Model file for the job. Use its own axes, mm. Face numbers are marked on the shaded views. A direction names the side the tool comes from. Round coordinates to 2 decimals unless told otherwise and drop trailing zeros. Order: outer loops, then holes, each group sorted by start corner. A loop starts at its lowest first (then second) coordinate and runs counter-clockwise, first axis right, second up. Notation, with made-up numbers: (18.25, 63) -> (38.25, 63) arc R12 cw to (38.25, 77) -> close; hole circle Ø4 at (20, 48). An arc over 180 degrees is marked (long way). Use CSV: the item, a comma, the result in double quotes.
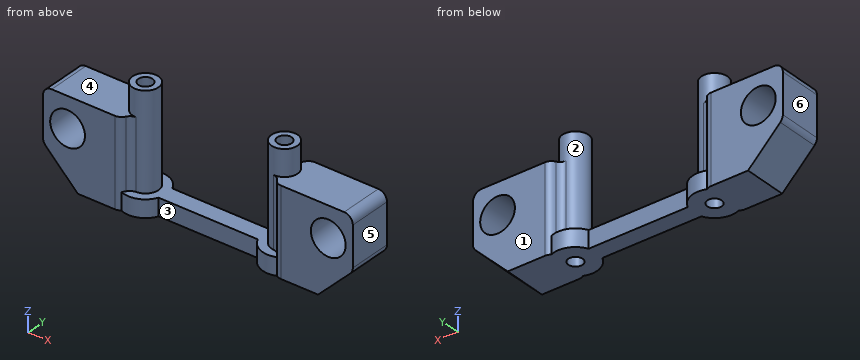
Autodesk Inventor part; units mm, degrees
ref_plane "YZ Plane" through (0, 0, 0) normal (1, 0, 0) x (0, 1, 0)
ref_plane "XZ Plane" through (0, 0, 0) normal (0, 1, 0) x (-1, 0, 0)
ref_plane "XY Plane" through (0, 0, 0) normal (0, 0, 1) x (1, 0, 0)
sketch "Sketch1" plane through (0, 0, 0) normal (0, 0, 1) x (1, 0, 0)
  circle A0 centre (0, 0) radius 1.65
  circle A1 centre (0, 0) radius 3
  circle A2 centre (32, 0) radius 1.65
  circle A3 centre (32, 0) radius 3
  dimension "d0" = 3.3
  dimension "d1" = 6
  dimension "d22" = 32
extrude "Extrusion1" add sketch "Sketch1" along normal blind 26
sketch "Sketch2" plane through (0, 0, 0) normal (0, 0, -1) x (-1, 0, 0)
  circle A0 centre (0, 0) radius 3
  circle A1 centre (0, 0) radius 5
  circle A2 centre (-32, 0) radius 1.65
  circle A3 centre (-32, 0) radius 5
  circle A4 centre (0, 0) radius 1.65 construction
  line L0 (-30.35, 2) -> (-1.65, 2)
  line L1 (-1.65, 2) -> (-1.65, -2)
  line L2 (-1.65, -2) -> (-30.35, -2)
  line L3 (-30.35, -2) -> (-30.35, 2)
  point P0 (-1.65, 0)
  dimension "d4" = 10
  dimension "d7" = 4
extrude "Extrusion2" add sketch "Sketch2" against normal blind 4 contours A0 L0 A1 L2 | L0 L1 L2 A0 | A0 L2 A1 L0 | A1 L2 A3 L0 | L0 L3 L2 A3 | A3 L2 L3 L0 picked at (-2.1, 0)
sketch "Sketch3" plane through (0, 0, 0) normal (0, 0, -1) x (-1, 0, 0)
  line L0 (-51.65, -5) -> (-33.65, -5)
  line L1 (-33.65, -5) -> (-33.65, 5)
  line L2 (-33.65, 5) -> (-51.65, 5)
  line L3 (-51.65, 5) -> (-51.65, -5)
  line L4 (1.65, 5) -> (19.65, 5)
  line L5 (19.65, 5) -> (19.65, -5)
  line L6 (19.65, -5) -> (1.65, -5)
  line L7 (1.65, -5) -> (1.65, 5)
  circle A0 centre (0, 0) radius 1.65 construction
  circle A1 centre (-32, 0) radius 1.65 construction
  arc A2 (-27.4174, 2) -> (-27.4174, -2) centre (-32, 0) ccw construction
  arc A3 (-4.5826, -2) -> (-4.5826, 2) centre (0, 0) ccw construction
  point P0 (-33.65, 0)
  point P1 (1.65, 0)
  dimension "d8" = 18
  dimension "d10" = 18
extrude "Extrusion3" add sketch "Sketch3" against normal blind 20
sketch "Sketch4" plane through (33.65, 5, 0) normal (0, 1, 0) x (1, 0, 0)
  circle A0 centre (-47.65, -13) radius 4
  circle A1 centre (12.35, -13) radius 4
  line L0 (-35.3, -20) -> (-53.3, -20)
  line L1 (18, -20) -> (0, -20)
  line L2 (-35.3, 0) -> (-53.3, 0)
  line L3 (18, 0) -> (18, -20)
  line L4 (-53.3, 0) -> (-53.3, -20)
  point P0 (-33.65, 0)
  point P1 (-44.3, -20)
  point P2 (9, -20)
  dimension "d13" = 8
  dimension "d14" = 8
  dimension "d15" = 13
  dimension "d23" = 60
  dimension "d24" = 5.65
  dimension "d25" = 5.65
extrude "Extrusion4" cut sketch "Sketch4" against normal blind 20
chamfer "Chamfer1" distance 8 angle 45 2 edges at (51.65, 0, 0) (-19.65, 0, 0)
fillet "Fillet1" radius 2 12 edges at (33.65, 2.5055, 12) (33.65, -2.5055, 12) (33.65, 5, 10) (-1.65, 2.5055, 12) (-1.65, -2.5055, 12) (-1.65, 5, 10) (-1.65, -5, 10) (33.65, -5, 10) (51.65, 0, 20) (51.65, 0, 8) (-19.65, 0, 8) (-19.65, 0, 20)
equation "\"d10\" = d8"
equation "\"d24\" = d25"
properties part number "spacer stepperM n rail"
Q1. Cut at D-D (z = 13). Give the cut face in (x, y).
From the geometry:
outline,"(-19.65, -5) -> (-18, -5) -> (-18, 5) -> (-19.65, 5) -> close; (-10, -5) -> (-3.12, -5) arc R2 ccw to (-1.39, -3.99) arc R2 cw to (0.21, -2.99) arc R3 ccw to (0.21, 2.99) arc R2 cw to (-1.39, 3.99) arc R2 ccw to (-3.12, 5) -> (-10, 5) -> close; (31.79, -2.99) arc R2 cw to (33.39, -3.99) arc R2 ccw to (35.12, -5) -> (42, -5) -> (42, 5) -> (35.12, 5) arc R2 ccw to (33.39, 3.99) arc R2 cw to (31.79, 2.99) arc R3 ccw to start; (50, -5) -> (51.65, -5) -> (51.65, 5) -> (50, 5) -> close; hole circle Ø3.3 at (0, 0); hole circle Ø3.3 at (32, 0)"
Q2. Which spindle directions (+Z, -Z, +X, -X, +Y, -Y) get a long thin tool onto all of the face, cutting with end or side? Do the marked faces 1 and 2. Say none if no direction does.
From the geometry:
face 1,"+Z, -Z, +X, -X, +Y"
face 2,"+Z"
Q3. Mould opens along X. For the marked faces 3, 4, 5 and 6 say: +X half, -X half, draft (parallel to the pull), parting line (faces both ways), or undercut.
From the geometry:
face 3,"undercut"
face 4,"draft"
face 5,"+X half"
face 6,"-X half"
Q4. Pin check, flat tips, straight feed: pin 1 (3 mm diameter, centred on x = 16.5, z = 2.5, fed in from +Y); pin 2 (3 mm diameter, centred on x = -12, y = 1.5, fed in from +Z); pin 3 (1.2 mm diameter, centred on x = 17.5, z = 2, fed in from -Y). Stop position of each tip, or through.
From the geometry:
pin 1,"stops at y = 2"
pin 2,"stops at z = 20"
pin 3,"stops at y = -2"
Q5. Probe line 1 along X through (y, z) = (2.5, 13); line 2 along X through (y, z) = (-0.75, 13); line 3 along X through (y, z) = (0.5, 21.5). List the from-to ranges inside material, lowest first.
From the geometry:
line 1,"x = -19.65 to -18, -10 to 1.66, 30.34 to 42, 50 to 51.65"
line 2,"x = -19.65 to -18, -10 to -1.47, 1.47 to 2.9, 29.1 to 30.53, 33.47 to 42, 50 to 51.65"
line 3,"x = -2.96 to -1.57, 1.57 to 2.96, 29.04 to 30.43, 33.57 to 34.96"
Q6. Cut at C-C (x = -14). Give the cut face in (y, z), plus the area to 3 significant figures.
From the geometry:
outline,"(-5, 2.35) -> (5, 2.35) -> (5, 9) -> (-5, 9) -> close; (-5, 17) -> (5, 17) -> (5, 20) -> (-5, 20) -> close"
area,"96.5 mm²"
Q7. Cut at A-A (y = 0). Give the cut face in (x, z), plus the area to 3 significant figures.
From the geometry:
outline,"(-19.65, 8.83) arc R2 ccw to (-19.06, 7.41) -> (-11.65, 0) -> (-1.65, 0) -> (-1.65, 26) -> (-3, 26) -> (-3, 20) -> (-17.65, 20) arc R2 ccw to (-19.65, 18) -> close; (1.65, 0) -> (30.35, 0) -> (30.35, 26) -> (29, 26) -> (29, 4) -> (3, 4) -> (3, 26) -> (1.65, 26) -> close; (33.65, 0) -> (43.65, 0) -> (51.06, 7.41) arc R2 ccw to (51.65, 8.83) -> (51.65, 18) arc R2 ccw to (49.65, 20) -> (35, 20) -> (35, 26) -> (33.65, 26) -> close; hole circle Ø8 at (-14, 13); hole circle Ø8 at (46, 13)"
area,"744 mm²"
Q8. Cut at B-B (z = 6.5). Give the cut face in (x, y).
From the geometry:
outline,"(-18.15, -5) -> (-3.12, -5) arc R2 ccw to (-1.39, -3.99) arc R2 cw to (0.21, -2.99) arc R3 ccw to (0.21, 2.99) arc R2 cw to (-1.39, 3.99) arc R2 ccw to (-3.12, 5) -> (-18.15, 5) -> close; (31.79, -2.99) arc R2 cw to (33.39, -3.99) arc R2 ccw to (35.12, -5) -> (50.15, -5) -> (50.15, 5) -> (35.12, 5) arc R2 ccw to (33.39, 3.99) arc R2 cw to (31.79, 2.99) arc R3 ccw to start; hole circle Ø3.3 at (0, 0); hole circle Ø3.3 at (32, 0)"
